```python
from build123d import *

# Parameters (mm, degrees)
SKETCH_W        = 50
SKETCH_H        = 52
PAD_DEPTH       = 21.5
SKETCH001_W     = 48
SKETCH001_H     = 50
POCKET_DEPTH    = 20.5
SKETCH002_W     = 6.5
SKETCH002_H     = 6.5
PAD001_DEPTH    = 4
SKETCH003_R     = 0.5
POCKET001_DEPTH = 3
SKETCH004_W     = 26.55
SKETCH004_H     = 15.5
POCKET002_DEPTH = 1
SKETCH005_W     = 10
SKETCH005_H     = 5
SKETCH005_W_2   = 16
SKETCH005_H_2   = 3
POCKET003_DEPTH = 1
SKETCH006_W     = 2
SKETCH006_H     = 5.5
POCKET004_DEPTH = 1
FILLET_R        = 1
SKETCH007_R     = 3.25
POCKET005_DEPTH = 1


with BuildPart() as part:
    # Sketch → Pad (new body)
    with BuildSketch(Plane.XY):
        Rectangle(SKETCH_W, SKETCH_H)
    extrude(amount=PAD_DEPTH)

    # Sketch001 (on Face6 of Pad) → Pocket (cut)
    with BuildSketch(Plane.XY.offset(21.5)):
        Rectangle(SKETCH001_W, SKETCH001_H)
    extrude(amount=-POCKET_DEPTH, mode=Mode.SUBTRACT)

    # Sketch002 (on Face11 of Pocket) → Pad001 (join)
    with BuildSketch(Plane.XY.offset(1)):
        with Locations((-20.75, 21.75)):
            Rectangle(SKETCH002_W, SKETCH002_H)
        with Locations((20.75, 21.75)):
            Rectangle(SKETCH002_W, SKETCH002_H)
        with Locations((-20.75, -21.75)):
            Rectangle(SKETCH002_W, SKETCH002_H)
        with Locations((20.75, -21.75)):
            Rectangle(SKETCH002_W, SKETCH002_H)
    extrude(amount=PAD001_DEPTH)

    # Sketch003 (on DatumPlane) → Pocket001 (cut)
    with BuildSketch(Plane.XY.offset(5)):
        with Locations((-20, 21)):
            Circle(SKETCH003_R)
        with Locations((20, 21)):
            Circle(SKETCH003_R)
        with Locations((-20, -21)):
            Circle(SKETCH003_R)
        with Locations((20, -21)):
            Circle(SKETCH003_R)
    extrude(amount=-POCKET001_DEPTH, mode=Mode.SUBTRACT)

    # Sketch004 (on Face6 of Pocket001) → Pocket002 (cut)
    with BuildSketch(Plane.XZ.offset(26)):
        with Locations((4.025, 13.75)):
            Rectangle(SKETCH004_W, SKETCH004_H)
    extrude(amount=-POCKET002_DEPTH, mode=Mode.SUBTRACT)

    # Sketch005 (on Face1 of Pocket002) → Pocket003 (cut)
    with BuildSketch(Plane(origin=(0, 26, 0), x_dir=(-1, 0, 0), z_dir=(0, 1, 0))):
        with Locations((-13, 8.5)):
            Rectangle(SKETCH005_W, SKETCH005_H)
        with Locations((4, 4)):
            Rectangle(SKETCH005_W_2, SKETCH005_H_2)
    extrude(amount=-POCKET003_DEPTH, mode=Mode.SUBTRACT)

    # Sketch006 → Pocket004 (cut)
    with BuildSketch(Plane.YZ.offset(25)):
        with Locations((17, 16.25)):
            Rectangle(SKETCH006_W, SKETCH006_H)
        with Locations((13, 16.25)):
            Rectangle(SKETCH006_W, SKETCH006_H)
        with Locations((9, 16.25)):
            Rectangle(SKETCH006_W, SKETCH006_H)
        with Locations((5, 16.25)):
            Rectangle(SKETCH006_W, SKETCH006_H)
        with Locations((5, 8.75)):
            Rectangle(SKETCH006_W, SKETCH006_H)
        with Locations((9, 8.75)):
            Rectangle(SKETCH006_W, SKETCH006_H)
        with Locations((13, 8.75)):
            Rectangle(SKETCH006_W, SKETCH006_H)
        with Locations((17, 8.75)):
            Rectangle(SKETCH006_W, SKETCH006_H)
    extrude(amount=-POCKET004_DEPTH, mode=Mode.SUBTRACT)

    # Fillet
    fillet_edges = [part.edges().sort_by_distance(p)[0] for p in [
        (-25, 0, 0),
        (0, -26, 0),
        (25, 0, 0),
        (0, 26, 0),
        (25, 26, 10.75),
        (25, -26, 10.75),
        (-25, -26, 10.75),
        (-25, 26, 10.75),
    ]]
    fillet(fillet_edges, radius=FILLET_R)

    # Sketch007 (on Face1 of Fillet) → Pocket005 (cut)
    with BuildSketch(Plane(origin=(0, 26, 0), x_dir=(-1, 0, 0), z_dir=(0, 1, 0))):
        with Locations((8, 14.5)):
            Circle(SKETCH007_R)
    extrude(amount=-POCKET005_DEPTH, mode=Mode.SUBTRACT)


solid = part.part
```
Work out the finished part from the listing and answer in its coordinate system (mm). A direction names the side the tool comes from. Give positions to 0.01 mm unless a question says otherwise; leave off trailing zeros. Loops run counter-clockwise (first coordinate to the right, second up) from the corner with the lowest first, then second, coordinate; pieces in that order, holes last. Notation, with made-up numbers: (44.5, 60.5) -> (78.5, 60.5) arc R22 cw to (78.5, 75.5) -> close; hole circle Ø10 at (84, 61.5). An arc over 180 degrees is marked (long way). Write item = value, one per line. Start each with the question number.
(1) Find the intervals of material crossed by probe 1 along Y at (x, z) = (20, 4.1); probe 2 along Y at (x, z) = (7.5, 4); probe 3 along Z at (x, y) = (-8, 25.5), in increasing order. Write a range as from..to.
(2) Find section C-C on y = -12.5. Give the vertices of the cut face in (x, z), and give its area (3 significant figures).
(3) The mould has two halves that part along Z. Classify faces 3 (the cylindrical face through (-5.605, 25.507, 16.697)), 4 (the flat face through (0, 0, 0)), 5 (the flat face through (21, 18.5, 3)), 6 (the flat face through (21, -22, 5)): +Z half, -Z half, draft (parallel to the pull), parting line (faces both ways), or undercut.
(4) Find section D-D on z = 8.5. Give the number of separate pieces and of enclosed holes in the cut face, and give its area (3 significant figures).
(5) Find section A-A on x = -8. Give the vertices of the cut face in (y, z), and give its area (3 significant figures).
(6) Given pin 1 Ø2 at (x, y) = (19.5, -20.5) entering from +Z; pin 2 Ø0.8 at (x, z) = (24.5, 9.5) entering from +Y (3 decimals); pin 3 Ø0.8 at (x, y) = (13.5, 25.5) entering from -Z (3 decimals), each flat-ended and moving along its own axis, determine where each tip first touches the part or whether it passes through.
(7) Find section B-B on x = -0.5. Give the vertices of the cut face in (y, z).
(8) Which of the six approach directions +Z, -Z, +X, -X, +Y, -Y give full straight-line access (tool end or side, diameter ignored) to faces 1 (the flat face through (17.5, 22, 3)), 2 (the flat face through (25, 0, 11))?
From the geometry:
q1.probe_1 = -26..-21.5, -20.5..-18.5, 18.5..20.5, 21.5..26
q1.probe_2 = -26..-25, 25..26
q1.probe_3 = 0.13..2.5, 5.5..11.25, 17.75..21.5
q2.outline = (-25, 1) arc R1 ccw to (-24, 0) -> (24, 0) arc R1 ccw to (25, 1) -> (25, 21.5) -> (24, 21.5) -> (24, 1) -> (-24, 1) -> (-24, 21.5) -> (-25, 21.5) -> close
q2.area = 90.6 mm^2
q3.face_3 = undercut
q3.face_4 = -Z half
q3.face_5 = draft
q3.face_6 = +Z half
q4.separate_pieces = 6
q4.enclosed_holes = 0
q4.area = 155 mm^2
q5.outline = (-26, 1) arc R1 ccw to (-25, 0) -> (25, 0) arc R1 ccw to (26, 1) -> (26, 2.5) -> (25, 2.5) -> (25, 1) -> (-25, 1) -> (-25, 6) -> (-26, 6) -> close; (25, 5.5) -> (26, 5.5) -> (26, 11.25) -> (25, 11.25) -> close; (25, 17.75) -> (26, 17.75) -> (26, 21.5) -> (25, 21.5) -> close
q5.area = 67.6 mm^2
q6.pin_1 = 5
q6.pin_2 = 25.995
q6.pin_3 = 0.005
q7.outline = (-26, 1) arc R1 ccw to (-25, 0) -> (25, 0) arc R1 ccw to (26, 1) -> (26, 2.5) -> (25, 2.5) -> (25, 1) -> (-25, 1) -> (-25, 6) -> (-26, 6) -> close; (25, 5.5) -> (26, 5.5) -> (26, 21.5) -> (25, 21.5) -> close
q8.face_1 = +Z
q8.face_2 = +Z, -Z, +X, +Y, -Y
